Autodesk Inventor part; units mm, degrees
ref_plane "YZ Plane" through (0, 0, 0) normal (1, 0, 0) x (0, 1, 0)
ref_plane "XZ Plane" through (0, 0, 0) normal (0, 1, 0) x (-1, 0, 0)
ref_plane "XY Plane" through (0, 0, 0) normal (0, 0, 1) x (1, 0, 0)
sketch "Skizze1" plane through (0, 0, 0) normal (1, 0, 0) x (0, 1, 0)
  line L0 (0, 0) -> (198, 0)
  line L1 (198, 0) -> (198, 92)
  line L2 (198, 92) -> (0, 92)
  line L3 (0, 92) -> (0, 0)
  dimension "d0" = 198
  dimension "d1" = 92
extrude "Extrusion1" add sketch "Skizze1" along normal blind 10
sketch "Skizze2" plane through (10, 0, 0) normal (1, 0, 0) x (0, 0, -1)
  line L0 (-92, 0) -> (0, 0)
  line L1 (-85.5, 147.5) -> (-85.5, 50.5) construction
  line L2 (0, 0) -> (0, 198)
  dimension "d4" = 97
  dimension "d5" = 50.5
  dimension "d6" = 85.5
hole "Bohrung1" at (10, 147.5, 85.5) at (10, 50.5, 85.5) direction (-1, 0, 0) diameter 4.2 depth 10
sketch "Skizze3" plane through (10, 0, 0) normal (1, 0, 0) x (0, 0, -1)
  circle A0 centre (-85.5, 147.5) radius 2.1
  circle A1 centre (-85.5, 50.5) radius 2.1
  arc A2 (-92, 50.5) -> (-89.052, 45.0563) centre (-85.5, 50.5) ccw
  arc A3 (-89.052, 152.9437) -> (-92, 147.5) centre (-85.5, 147.5) ccw
  line L0 (0, 0) -> (0, 198)
  line L1 (0, 198) -> (-20, 198) construction
  line L2 (0, 0) -> (-20, 0) construction
  line L3 (-92, 0) -> (0, 0)
  line L4 (-20, 0) -> (-89.052, 45.0563)
  line L5 (-20, 198) -> (-89.052, 152.9437)
  line L6 (-92, 198) -> (-92, 0)
  line L7 (-20, 198) -> (-92, 198)
  line L8 (-92, 147.5) -> (-92, 198)
  line L9 (-92, 50.5) -> (-92, 0)
  line L10 (-92, 0) -> (-20, 0)
  dimension "d15" = 20
extrude "Extrusion2" cut sketch "Skizze3" against normal up to surface (10 mm away) contours L6 L7 L5 A3 | A2 L4 L3 L6
sketch "Skizze4" plane through (10, 0, 0) normal (1, 0, 0) x (0, 0, -1)
  line L0 (0, 0) -> (0, 198)
  line L1 (-20, 0) -> (0, 0)
  line L2 (0, 198) -> (-20, 198)
  line L3 (-92, 147.5) -> (-92, 50.5)
  line L4 (-92, 99) -> (0, 99)
  point P0 (-10, 10)
  point P1 (-10, 188)
  point P2 (-10, 99)
  dimension "d18" = 10
  dimension "d19" = 10
  dimension "d20" = 10
hole "Bohrung2" at (10, 10, 10) at (10, 188, 10) at (10, 99, 10) direction (-1, 0, 0) diameter 4.5 end through all counterbore diameter 8 counterbore depth 5
fillet "Rundung1" radius 5 4 edges at (5, 198, 20) (5, 0, 20) (5, 0, 0) (5, 198, 0)
properties part number "102.006.01_Anbindung_Aktor"
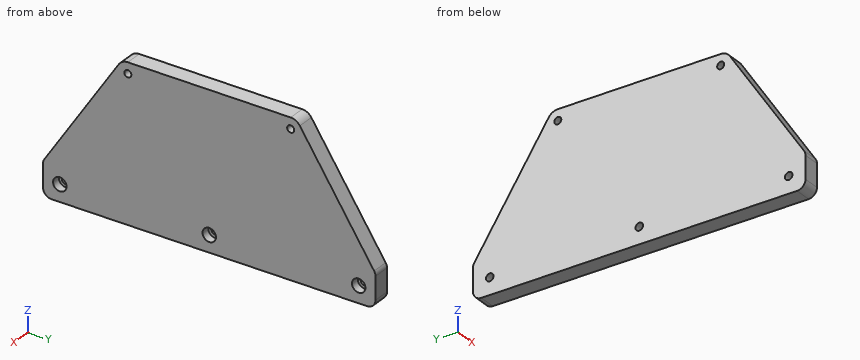
Model file for the job. Use its own axes, mm. Round coordinates to 2 decimals unless told otherwise and drop trailing zeros. Order: outer loops, then holes, each group sorted by start corner. A loop starts at its lowest first (then second) coordinate and runs counter-clockwise, first axis right, second up. Notation, with made-up numbers: (0.5, -34.75) -> (31.5, -34.75) arc R36 ccw to (31.5, -0.75) -> close; hole circle Ø3 at (-12, 12.5). An arc over 180 degrees is marked (long way). Use one line per item in the form item = value.
Item 1: Drill centre lines: line 1 (Y direction, x = 3.1, z = 10); line 2 (Y direction, x = 7.7, z = 10); line 3 (Z direction, x = 2.05, y = 99). Where is each one in solid material? Low to high.
Returned:
line_1 = 0 to 7.75, 12.25 to 96.75, 101.25 to 185.75, 190.25 to 198
line_2 = 0 to 6, 14 to 95, 103 to 184, 192 to 198
line_3 = 0 to 7.75, 12.25 to 92
Item 2: Cut at C-C, the plane x = 3. Write the cut outline in (y, z).
Returned:
outline = (0, 5) arc R5 ccw to (5, 0) -> (193, 0) arc R5 ccw to (198, 5) -> (198, 18.51) arc R5 ccw to (197.19, 21.25) -> (152.94, 89.05) arc R6.5 ccw to (147.5, 92) -> (50.5, 92) arc R6.5 ccw to (45.06, 89.05) -> (0.81, 21.25) arc R5 ccw to (0, 18.51) -> close; hole circle Ø4.5 at (10, 10); hole circle Ø4.2 at (50.5, 85.5); hole circle Ø4.5 at (99, 10); hole circle Ø4.2 at (147.5, 85.5); hole circle Ø4.5 at (188, 10)
Item 3: Flat gauge pins, fed straight in: pin 1 Ø7 at (y, z) = (99, 10) entering from +X; pin 2 Ø6 at (x, z) = (3.5, 33) entering from -Y (3 decimals); pin 3 Ø5 at (x, z) = (5, 38.5) entering from -Y. Where does each tip first touch, or does it go through?
Returned:
pin_1 = 5
pin_2 = 6.525
pin_3 = 10.44
Item 4: Cut at B-B, the plane z = 10. Write the cut outline in (x, y), and give its area (3 significant figures).
Returned:
outline = (0, 0) -> (10, 0) -> (10, 6) -> (5, 6) -> (5, 7.75) -> (0, 7.75) -> close; (0, 12.25) -> (5, 12.25) -> (5, 14) -> (10, 14) -> (10, 95) -> (5, 95) -> (5, 96.75) -> (0, 96.75) -> close; (0, 101.25) -> (5, 101.25) -> (5, 103) -> (10, 103) -> (10, 184) -> (5, 184) -> (5, 185.75) -> (0, 185.75) -> close; (0, 190.25) -> (5, 190.25) -> (5, 192) -> (10, 192) -> (10, 198) -> (0, 198) -> close
area = 1,790 mm^2
Item 5: Cut at A-A, the plane y = 99. Write the cut outline in (x, z).
Returned:
outline = (0, 0) -> (10, 0) -> (10, 6) -> (5, 6) -> (5, 7.75) -> (0, 7.75) -> close; (0, 12.25) -> (5, 12.25) -> (5, 14) -> (10, 14) -> (10, 92) -> (0, 92) -> close
Item 6: Cut at D-D, the plane z = 85.5. Write the cut outline in (x, y), and give its area (3 significant figures).
Returned:
outline = (0, 42.74) -> (10, 42.74) -> (10, 48.4) -> (0, 48.4) -> close; (0, 52.6) -> (10, 52.6) -> (10, 145.4) -> (0, 145.4) -> close; (0, 149.6) -> (10, 149.6) -> (10, 155.26) -> (0, 155.26) -> close
area = 1,040 mm^2
